Work out the finished part from the listing and answer in its coordinate system (mm). A direction names the side the tool comes from. Coordinates: 2 decimals unless noted, no trailing zeros. Loops run counter-clockwise (first coordinate to the right, second up) from the corner with the lowest first, then second, coordinate; pieces in that order, holes last. Notation, with made-up numbers: (83, -0.75) -> (131, -0.75) arc R28 cw to (131, 29.25) -> close; hole circle Ø10 at (71, -29.5). An arc over 180 degrees is marked (long way). Answer as CSV lines item,"result".
```python
from build123d import *

# Parameters (mm, degrees)
SKETCH1_W           = 533.4
SKETCH1_H           = 2.54
BOSS_EXTRUDE1_DEPTH = 203.2
FILLET1_R           = 2.54
SKETCH3_R           = 3.175
BOSS_EXTRUDE2_DEPTH = 101.6
SKETCH5_R           = 1.905
BOSS_EXTRUDE3_DEPTH = 25.4
BOSS_EXTRUDE4_START = 25.4
SKETCH6_R           = 1.905
BOSS_EXTRUDE4_DEPTH = 25.4


with BuildPart() as part:
    # Sketch1 → Boss-Extrude1 (new body)
    with BuildSketch(Plane.XY):
        Rectangle(SKETCH1_W, SKETCH1_H)
    extrude(amount=BOSS_EXTRUDE1_DEPTH)

    # Fillet1
    fillet1_edges = [part.edges().sort_by_distance(p)[0] for p in [
        (-266.7, 0, 203.2),
        (266.7, 0, 203.2),
        (-266.7, 0, 0),
        (266.7, 0, 0),
    ]]
    fillet(fillet1_edges, radius=FILLET1_R)

    # Sketch3 → Boss-Extrude2 (add)
    with BuildSketch(Plane.ZY.offset(50.8)):
        with BuildLine():
            ThreePointArc((-0.875862069, 2.189655172), (-0.227086506, 1.179165397), (0, 0))
            Line((0, 0), (0, 1.27))
            Line((0, 1.27), (-0.875862069, 2.189655172))
        make_face()
        with BuildLine():
            Line((-0.875862069, -2.189655172), (0, -1.27))
            Line((0, -1.27), (0, 0))
            ThreePointArc((0, 0), (-0.227086506, -1.179165397), (-0.875862069, -2.189655172))
        make_face()
        with Locations((-3.175, 0)):
            Circle(SKETCH3_R)
    extrude(amount=-BOSS_EXTRUDE2_DEPTH)

    # Sketch5 → Boss-Extrude3 (add)
    with BuildSketch(Plane.ZY.offset(50.8)):
        with Locations((-3.175, 0)):
            Circle(SKETCH5_R)
    extrude(amount=BOSS_EXTRUDE3_DEPTH)

    # Sketch6 → Boss-Extrude4 (add)
    with BuildSketch(Plane(origin=(50.8, 0, 0), x_dir=(0, 0, -1), z_dir=(1, 0, 0)).offset(BOSS_EXTRUDE4_START)):
        with Locations(Location((3.175, 0, 0), (0, 0, 180))):
            Circle(SKETCH6_R)
    extrude(amount=-BOSS_EXTRUDE4_DEPTH)


solid = part.part
```
(1) Consider line 1 along Y through (x, z) = (53.5, 2); line 2 along Z through (x, y) = (-24, -0.75); line 3 along Z through (x, y) = (-55, 0.5). Determine where each line is inside the solid, lowest interval first.
Computed values:
line 1,"-1.27 to 1.27"
line 2,"-6.26 to 203.2"
line 3,"-5.01 to -1.34, 0 to 203.2"
(2) Which of the six approach directions +Z, -Z, +X, -X, +Y, -Y give full straight-line access (tool end or side, diameter ignored) to faces 1 (the face through (-4, -1.27, 100)), 2 (the face through (-4, 1.27, 100))?
Computed values:
face 1,"+Z, +X, -X, -Y"
face 2,"+Z, +X, -X, +Y"
(3) A cutting plane is placed at A-A, the plane y = 0. Write down the section's boundary in (x, z).
Computed values:
outline,"(-266.7, 2.54) arc R2.54 ccw to (-264.16, 0) -> (-50.8, 0) -> (-50.8, -1.27) -> (-76.2, -1.27) -> (-76.2, -5.08) -> (-50.8, -5.08) -> (-50.8, -6.35) -> (50.8, -6.35) -> (50.8, -5.08) -> (76.2, -5.08) -> (76.2, -1.27) -> (50.8, -1.27) -> (50.8, 0) -> (264.16, 0) arc R2.54 ccw to (266.7, 2.54) -> (266.7, 200.66) arc R2.54 ccw to (264.16, 203.2) -> (-264.16, 203.2) arc R2.54 ccw to (-266.7, 200.66) -> close"
(4) A cutting plane is placed at C-C, the plane x = -93. Write down the section's boundary in (y, z).
Computed values:
outline,"(-1.27, 0) -> (1.27, 0) -> (1.27, 203.2) -> (-1.27, 203.2) -> close"
(5) Flat-ended cylindrical pins translate along their axes: pin 1 Ø8 at (x, z) = (44, 51) entering from -Y; pin 2 Ø4 at (x, z) = (-23.5, 60) entering from +Y; pin 3 Ø0.8 at (x, y) = (115, 0.5) entering from -Z. Find the tip coordinate at first contact, or state that the pin passes through.
Computed values:
pin 1,"y = -1.27"
pin 2,"y = 1.27"
pin 3,"z = 0"
(6) A cutting plane is placed at B-B, the plane z = 129. Write down the section's boundary in (x, y), and give its area (3 significant figures).
Computed values:
outline,"(-266.7, -1.27) -> (266.7, -1.27) -> (266.7, 1.27) -> (-266.7, 1.27) -> close"
area,"1,350 mm2"
